Source: CAD feature listing. Evaluate the final solid. Frame: model axes, mm. A direction names the side the tool comes from. Give positions to 0.01 mm unless a question says otherwise; leave off trailing zeros. Order: outer loops, then holes, each group sorted by start corner. A loop starts at its lowest first (then second) coordinate and runs counter-clockwise, first axis right, second up. Notation, with made-up numbers: M 65.5,7 L 91.5,7 A15 cw 91.5,34 Z; hole C 53,19.5 d7. An arc over 180 degrees is marked long. Answer as a JSON object with one key per item and string values. Group by question number.
1. Pull-direction query (X, two-part tool) for faces 3 (the flat face through (-86, 47, 10)), 4 (the flat face through (-97.36, 6.32, 2.46)), 5 (the flat face through (-93, 30, 0)); classes: +X half, -X half, draft (parallel to the pull), parting line (faces both ways), or undercut.
2. Set-up query: faces 1 (the flat face through (-94, 26, 10)), 2 (the flat face through (-82.58, 51.71, 10.85)). Return all of +Z, -Z, +X, -X, +Y, -Y with unobstructed straight access to the full face (end or side cutting, diameter ignored); none if empty.
3. Section query C-C (y = 11). Output: boundary loops of the cut face in (x, z).
4. Section query B-B (x = -93.25). Output: boundary loops of the cut face in (y, z), plus the area to 3 significant figures.
5. Pin query (flat end, axial travel): P1, Ø3, axis at x = -90, z = 11.5, coming from the +Y side; P2, Ø2, axis at y = 33.5, z = 10.5, coming from the -X side; P3, Ø1.5, axis at x = -94, y = 25.5, coming from the -Z side. Return the tip coordinate at first contact, or that it passes through.
6. Material intervals for L1, parallel to X at y = 46.5, z = 3.5; L2, parallel to X at y = 15.5, z = 2; L3, parallel to X at y = 24.5, z = 3.25, sorted ascending. Write a range as [from, to].
7. Section query A-A (z = 7.5). Output: boundary loops of the cut face in (x, y), plus the area to 3 significant figures.
8. Section query D-D (z = 16). Output: boundary loops of the cut face in (x, y).
from build123d import *

# Parameters (mm, degrees)
F0_R        = 1.5
F1_DEPTH    = 22
F2_T1_DEPTH = 165.5952281179
F3_DEPTH    = 10


# Not quite as in the source:
# - a fillet or chamfer that OpenCascade refuses, or shapes differently, is made with other operations: its cross-section is extruded or revolved along the edge and cut away or added


with BuildPart() as f1:
    # F0 (on Top) → F1 (new body)
    with BuildSketch(Plane.XY):
        with BuildLine():
            ThreePointArc((-92.2088082298, 7.3338724312), (-92.0714667591, 8.8935374755), (-91.9077462525, 10.4506544671))
            Line((-91.9077462525, 10.4506544671), (-102.1523712509, 8.4346338282))
            ThreePointArc((-102.1523712509, 8.4346338282), (-102.2684274731, 6.8861267905), (-102.3610115463, 5.3360392827))
            Line((-102.3610115463, 5.3360392827), (-92.2088082298, 7.3338724312))
        make_face()
        with BuildLine():
            ThreePointArc((-91.5835416646, 12.9886448933), (-87.4986604127, 30.0039068455), (-80.2824351959, 45.9454089003))
            Line((-80.2824351959, 45.9454089003), (-88.9616173792, 50.9124801328))
            ThreePointArc((-88.9616173792, 50.9124801328), (-96.9579750519, 33.2475724504), (-101.4844650878, 14.3928227196))
            Line((-101.4844650878, 14.3928227196), (-91.5835416646, 12.9886448933))
        make_face()
        with Locations((-94.0054339813, 25.8694488148)):
            Circle(F0_R, mode=Mode.SUBTRACT)
        with Locations((-85.5445299814, 46.7801602206)):
            Circle(F0_R, mode=Mode.SUBTRACT)
        with BuildLine():
            ThreePointArc((-80.2824351959, 45.9454089003), (-79.3561481615, 47.5273789407), (-78.3986924261, 49.0906816603))
            Line((-78.3986924261, 49.0906816603), (-86.8742267425, 54.3977823804))
            ThreePointArc((-86.8742267425, 54.3977823804), (-87.935191206, 52.6654739613), (-88.9616173792, 50.9124801328))
            Line((-88.9616173792, 50.9124801328), (-80.2824351959, 45.9454089003))
        make_face()
        with BuildLine():
            ThreePointArc((-91.9077462525, 10.4506544671), (-91.7544196986, 11.720770699), (-91.5835416646, 12.9886448933))
            Line((-91.5835416646, 12.9886448933), (-101.4844650878, 14.3928227196))
            ThreePointArc((-101.4844650878, 14.3928227196), (-101.8619913522, 11.4186127778), (-102.1523712509, 8.4346338282))
            Line((-102.1523712509, 8.4346338282), (-91.9077462525, 10.4506544671))
        make_face()
        with Locations((-85.5445299814, 46.7801602206)):
            Circle(F0_R)
        with Locations((-94.0054339813, 25.8694488148)):
            Circle(F0_R)
    extrude(amount=F1_DEPTH)

    # F2: chamfer of 17 x 30 on 1 edges, made by hand

    # F2_s2 → F2_t1 (cut)
    with BuildSketch(Plane(origin=(-173.6973169445, -34.1815709152, 0), x_dir=(0, 0, 1), z_dir=(0.9811820369, 0.1930849823, 0))):
        Polygon((5, -25), (22, -55), (22, -25), align=None)
    extrude(amount=F2_T1_DEPTH, mode=Mode.SUBTRACT)

    # F0 (on Top) → F3 (cut)
    with BuildSketch(Plane.XY):
        with Locations((-85.5445299814, 46.7801602206)):
            Circle(F0_R)
        with Locations((-94.0054339813, 25.8694488148)):
            Circle(F0_R)
    extrude(amount=F3_DEPTH, mode=Mode.SUBTRACT)


solid = f1.part
Answer sheet:
{
 "1": {"face 3": "undercut", "face 4": "+X half", "face 5": "draft"},
 "2": {"face 1": "-Z", "face 2": "+Z, -Z, +X, +Y"},
 "3": {"outline": "M -101.91,0 L -91.84,0 L -91.84,7 L -101.91,8.1 Z"},
 "4": {"outline": "M 7.13,0 L 24.57,0 L 24.57,10 L 27.17,10 L 27.17,0 L 42.55,0 L 42.55,22 L 37.7,22 L 7.13,5 Z", "area": "494 mm^2"},
 "5": {"P1": "y = 51.71", "P2": "x = -97.21", "P3": "z = 10"},
 "6": {"L1": "[-91.35, -87.02], [-84.07, -79.96]", "L2": "[-101.32, -91.19]", "L3": "[-99.53, -94.62], [-93.39, -89.2]"},
 "7": {"outline": "M -102.02,9.9 L -91.73,11.92 A92.5 cw -78.4,49.09 L -86.87,54.4 A102.5 ccw Z; hole C -94.01,25.87 d3; hole C -85.54,46.78 d3", "area": "422 mm^2"},
 "8": {"outline": "M -99.22,25.74 L -88.19,27.91 A92.5 cw -78.4,49.09 L -86.87,54.4 A102.5 ccw Z"}
}
